```python
from build123d import *

# Parameters (mm, degrees)
F0_W     = 3.175
F0_H     = 6.35
F1_DEPTH = 3.175


with BuildPart() as f1:
    # F0 (on Top) → F1 (new body)
    with BuildSketch(Plane.XY):
        Polygon((-39.248684, 94.540516), (-44.963684, 94.540516), (-44.963684, 85.650516), (-44.963684, 79.300516), (-44.963684, 75.795316), (-44.963684, 69.445316), (-44.963684, 51.843116), (-44.963684, 45.493116), (-44.963684, 43.740516), (50.286316, 43.740516), (50.286316, 45.493116), (50.286316, 51.843116), (50.286316, 69.445316), (50.286316, 75.795316), (50.286316, 79.300516), (50.286316, 85.650516), (50.286316, 94.540516), (44.571316, 94.540516), (44.571316, 91.365516), (38.221316, 91.365516), (38.221316, 86.920516), (40.437466, 86.920516), (40.437466, 84.142391), (38.221316, 84.142391), (38.221316, 81.840516), (34.716116, 81.840516), (34.716116, 84.142391), (32.499966, 84.142391), (32.499966, 86.920516), (34.716116, 86.920516), (34.716116, 91.365516), (28.366116, 91.365516), (28.366116, 94.540516), (10.763916, 94.540516), (10.763916, 91.365516), (4.413916, 91.365516), (4.413916, 86.920516), (6.630066, 86.920516), (6.630066, 84.142391), (4.413916, 84.142391), (4.413916, 81.840516), (0.908716, 81.840516), (0.908716, 84.142391), (-1.307434, 84.142391), (-1.307434, 86.920516), (0.908716, 86.920516), (0.908716, 91.365516), (-5.441284, 91.365516), (-5.441284, 94.540516), (-23.043484, 94.540516), (-23.043484, 91.365516), (-29.393484, 91.365516), (-29.393484, 86.920516), (-27.177334, 86.920516), (-27.177334, 84.142391), (-29.393484, 84.142391), (-29.393484, 81.840516), (-32.898684, 81.840516), (-32.898684, 84.142391), (-35.114834, 84.142391), (-35.114834, 86.920516), (-32.898684, 86.920516), (-32.898684, 91.365516), (-39.248684, 91.365516), align=None)
        Polygon((50.286316, 43.740516), (-44.963684, 43.740516), (-44.963684, 41.987916), (-44.963684, 35.637916), (-44.963684, 18.035716), (-44.963684, 11.685716), (-44.963684, 8.180516), (-44.963684, 1.830516), (-44.963684, -7.059484), (-39.248684, -7.059484), (-39.248684, -3.884484), (-32.898684, -3.884484), (-32.898684, 0.560516), (-35.114834, 0.560516), (-35.114834, 3.338641), (-32.898684, 3.338641), (-32.898684, 5.640516), (-29.393484, 5.640516), (-29.393484, 3.338641), (-27.177334, 3.338641), (-27.177334, 0.560516), (-29.393484, 0.560516), (-29.393484, -3.884484), (-23.043484, -3.884484), (-23.043484, -7.059484), (-5.441284, -7.059484), (-5.441284, -3.884484), (0.908716, -3.884484), (0.908716, 0.560516), (-1.307434, 0.560516), (-1.307434, 3.338641), (0.908716, 3.338641), (0.908716, 5.640516), (4.413916, 5.640516), (4.413916, 3.338641), (6.630066, 3.338641), (6.630066, 0.560516), (4.413916, 0.560516), (4.413916, -3.884484), (10.763916, -3.884484), (10.763916, -7.059484), (28.366116, -7.059484), (28.366116, -3.884484), (34.716116, -3.884484), (34.716116, 0.560516), (32.499966, 0.560516), (32.499966, 3.338641), (34.716116, 3.338641), (34.716116, 5.640516), (38.221316, 5.640516), (38.221316, 3.338641), (40.437466, 3.338641), (40.437466, 0.560516), (38.221316, 0.560516), (38.221316, -3.884484), (44.571316, -3.884484), (44.571316, -7.059484), (50.286316, -7.059484), (50.286316, 1.830516), (50.286316, 8.180516), (50.286316, 11.685716), (50.286316, 18.035716), (50.286316, 35.637916), (50.286316, 41.987916), align=None)
        with Locations((-46.551184, 48.668116)):
            Rectangle(F0_W, F0_H)
        with Locations((-46.551184, 72.620316)):
            Rectangle(F0_W, F0_H)
        with Locations((-46.551184, 82.475516)):
            Rectangle(F0_W, F0_H)
        with Locations((-46.551184, 38.812916)):
            Rectangle(F0_W, F0_H)
        with Locations((-46.551184, 14.860716)):
            Rectangle(F0_W, F0_H)
        with Locations((-46.551184, 5.005516)):
            Rectangle(F0_W, F0_H)
        with Locations((51.873816, 5.005516)):
            Rectangle(F0_W, F0_H)
        with Locations((51.873816, 14.860716)):
            Rectangle(F0_W, F0_H)
        with Locations((51.873816, 38.812916)):
            Rectangle(F0_W, F0_H)
        with Locations((51.873816, 48.668116)):
            Rectangle(F0_W, F0_H)
        with Locations((51.873816, 72.620316)):
            Rectangle(F0_W, F0_H)
        with Locations((51.873816, 82.475516)):
            Rectangle(F0_W, F0_H)
    extrude(amount=F1_DEPTH)


solid = f1.part
```
For this review, take the finished solid that the model builds, in its own axes (mm). A direction names the side the tool comes from. Give positions to 0.01 mm unless a question says otherwise; leave off trailing zeros. Order: outer loops, then holes, each group sorted by start corner. A loop starts at its lowest first (then second) coordinate and runs counter-clockwise, first axis right, second up.
1) Insertion check: pin 1 (0.7 mm diameter, centred on x = -28, z = 1, fed in from -Y); pin 2 (1.8 mm diameter, centred on x = 34, z = 2, fed in from +Y); pin 3 (1.6 mm diameter, centred on y = 89.5, z = 2, fed in from -X). Each pin has a flat end and moves straight along its axis. Give the tip position at first contact, or say it passes through.
2) Wall thickness on line 1 (Y direction, x = 5.5, z = 1.95); line 2 (X direction, y = 11.5, z = 2.95); line 3 (Y direction, x = 3, z = 1.8): over which ranges is each line inside the solid? List them lowest first.
3) For faces 1 (the face through (36, 5.641, 2)), 2 (the face through (50.286, 10, 2)), 3 (the face through (6, 3.339, 2)), list the 3-axis set-ups (+Z, -Z, +X, -X, +Y, -Y) from which the entire face can be reached by the end or side of a thin tool; tool diameter is ignored.
4) Take a section at A-A (x = 9). Give the boundary of the cut face in (y, z) (3 decimals), then the cut area to 3 significant figures.
5) The part is to be moulded in two halves that separate along X. For faces 4 (the face through (52, 1.831, 2)), 5 (the face through (41, -3.884, 2)), 6 (the face through (-44.964, 27, 2)), 7 (the face through (50.286, 27, 2)), say which applies: released by +X, released by -X, zero draft, split by the parting line, or undercut.
Derived:
1. pin 1: stops at y = -3.88
1. pin 2: stops at y = 91.37
1. pin 3: stops at x = -44.96
2. line 1: y = -3.88 to 0.56, 3.34 to 84.14, 86.92 to 91.37
2. line 2: x = -44.96 to 50.29
2. line 3: y = 5.64 to 81.84
3. face 1: +Z, -Z, -Y
3. face 2: +Z, -Z, +X
3. face 3: +Z, -Z
4. outline: (-3.884, 0) - (91.366, 0) - (91.366, 3.175) - (-3.884, 3.175) - close
4. area: 302 mm2
5. face 4: zero draft
5. face 5: undercut
5. face 6: released by -X
5. face 7: released by +X
